from build123d import *

# Parameters (mm, degrees)
BOSS_EXTRUDE2_DEPTH = 110
BOSS_EXTRUDE4_DEPTH = 3
LPATTERN1_COUNT     = 17
LPATTERN1_PITCH     = 6


with BuildPart() as part:
    # Sketch1 → Boss-Extrude2 (new body)
    with BuildSketch(Plane(origin=(0, 0, 0), x_dir=(1, 0, 0), z_dir=(0, 1, 0))):
        with BuildLine():
            Line((25, 0), (40, 0))
            Line((40, 0), (40, 55))
            ThreePointArc((40, 55), (37.071067812, 62.071067812), (30, 65))
            Line((30, 65), (-30, 65))
            ThreePointArc((-30, 65), (-37.071067812, 62.071067812), (-40, 55))
            Line((-40, 55), (-40, 0))
            Line((-40, 0), (-25, 0))
            ThreePointArc((-25, 0), (0, 25), (25, 0))
        make_face()
    extrude(amount=BOSS_EXTRUDE2_DEPTH)

    # Sketch3 → Boss-Extrude4 (add)
    with BuildSketch(Plane.XZ):
        with BuildLine():
            Line((-44, 0), (-44, -55))
            ThreePointArc((-44, -55), (-39.899494937, -64.899494937), (-30, -69))
            Line((-30, -69), (30, -69))
            ThreePointArc((30, -69), (39.899494937, -64.899494937), (44, -55))
            Line((44, -55), (44, 0))
            Line((44, 0), (40, 0))
            Line((40, 0), (40, -55))
            ThreePointArc((40, -55), (37.071067812, -62.071067812), (30, -65))
            Line((30, -65), (-30, -65))
            ThreePointArc((-30, -65), (-37.071067812, -62.071067812), (-40, -55))
            Line((-40, -55), (-40, 0))
            Line((-40, 0), (-44, 0))
        make_face()
    boss_extrude4 = extrude(amount=-BOSS_EXTRUDE4_DEPTH)

    # LPattern1: Boss-Extrude4 ×17
    with Locations(*[(0, i * LPATTERN1_PITCH, 0) for i in range(1, LPATTERN1_COUNT)]):
        add(boss_extrude4)


solid = part.part
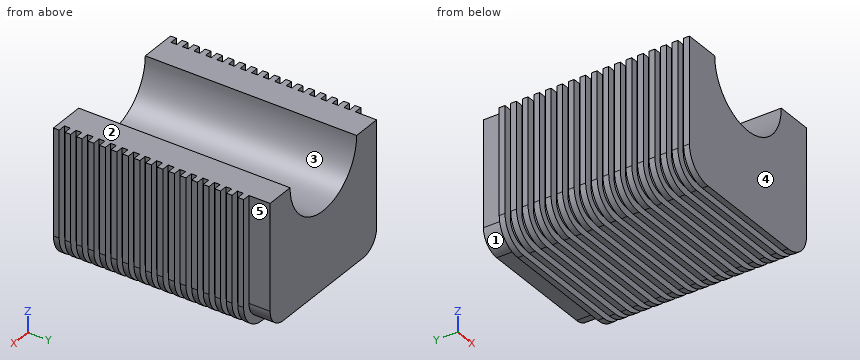
For this review, take the finished solid that the model builds, in its own axes (mm). Face numbers are marked on the shaded views. A direction names the side the tool comes from. Give positions to 0.01 mm unless a question says otherwise; leave off trailing zeros. Answer in a Markdown table with one row per item. Add a question column.
(1) Mouldability with a two-part tool opening along X and no side actions: class the marked faces 3, 4 and 5 as +X half, -X half, draft (parallel to the pull), parting line (faces both ways), or undercut.
(2) For pin 1 (10 mm diameter, centred on x = -23, y = 64.5, fed in from +Z); pin 2 (1.5 mm diameter, centred on y = 83, z = -24, fed in from -X); pin 3 (0.9 mm diameter, centred on y = 40, z = -32.5, fed in from +X); pin 4 (12 mm diameter, centred on x = -9, z = -11.5, fed in from -Y), all flat-tipped, find the tip position at first contact; note any pin that passes through.
(3) For the marked faces 1 and 2, list the 3-axis set-ups (+Z, -Z, +X, -X, +Y, -Y) from which the entire face can be reached by the end or side of a thin tool; tool diameter is ignored.
(4) Wall thickness on probe 1 along Z at (x, y) = (26, 102.5); probe 2 along X at (y, z) = (83, -50); probe 3 along X at (y, z) = (101, -4.5): over which ranges is each line inside the solid? List them lowest first. Write a range as [from, to].
Evaluation:
| question | item | result |
|---|---|---|
| 1 | face 3 | undercut |
| 1 | face 4 | draft |
| 1 | face 5 | +X half |
| 2 | pin 1 | stops at z = 0 |
| 2 | pin 2 | stops at x = -40 |
| 2 | pin 3 | stops at x = 40 |
| 2 | pin 4 | passes through |
| 3 | face 1 | -Z, -X, +Y |
| 3 | face 2 | +Z, +X, -X, +Y, -Y |
| 4 | probe 1 | z = [-65, 0] |
| 4 | probe 2 | x = [-40, 40] |
| 4 | probe 3 | x = [-40, -24.59], [24.59, 40] |
